Check sheet for the modelled part. Datum: model origin and axes. Units: mm. Round coordinates to 2 decimals unless told otherwise and drop trailing zeros. Order: outer loops, then holes, each group sorted by start corner. A loop starts at its lowest first (then second) coordinate and runs counter-clockwise, first axis right, second up. Notation, with made-up numbers: (17.25, 3.25) -> (41.25, 3.25) arc R13 cw to (41.25, 26.25) -> close; hole circle Ø3 at (16.5, 65.25). An arc over 180 degrees is marked (long way). Answer in a Markdown table with one row per item. Add a question column.
1. Depth check by flat-ended pin: P1, Ø3, axis at x = 75, z = -47, coming from the -Y side; P2, Ø1.1, axis at x = 21, y = 0.5, coming from the +Z side; P3, Ø1.1, axis at y = 0.5, z = -68, coming from the -X side; P4, Ø2.5, axis at x = -7.63, z = 0, coming from the +Y side. Enter the tip coordinate at first touch or a pass-through.
2. Material ranges on L1, parallel to X at y = 0.85, z = 0; L2, parallel to Y at x = 58, z = -13; L3, parallel to X at y = 0.4, z = 32.5, recorded low to high. Write a range as from..to.
3. Sectioned sample at A-A, the plane y = -6.5. Record the boundary of the cut face in (x, z).
4. Sectioned sample at C-C, the plane z = 24. Record the boundary of the cut face in (x, y), then the cut area to 3 significant figures.
5. Sectioned sample at B-B, the plane x = -84. Record the boundary of the cut face in (y, z).
```python
from build123d import *

# Parameters (mm, degrees)
SKETCH1_W            = 208
SKETCH1_H            = 147
BOSS_EXTRUDE1_DEPTH  = 1
CUT_EXTRUDE1_DEPTH   = 128.354819304
MIRROR2_COPY_1_DEPTH = 128.354819304
FILLET1_R            = 10
CUT_EXTRUDE2_DEPTH   = 128.354819304
SKETCH7_R            = 1.5
CUT_EXTRUDE3_DEPTH   = 128.354819304
SKETCH8_R            = 3
BOSS_EXTRUDE3_DEPTH  = 35
SKETCH9_R            = 1.4
CUT_EXTRUDE4_DEPTH   = 60


with BuildPart() as part:
    # Sketch1 → Boss-Extrude1 (new body)
    with BuildSketch(Plane(origin=(0, 0, 0), x_dir=(1, 0, 0), z_dir=(0, 1, 0))):
        Rectangle(SKETCH1_W, SKETCH1_H)
    extrude(amount=BOSS_EXTRUDE1_DEPTH)

    # Sketch3 → Cut-Extrude1 (cut, through all)
    with BuildSketch(Plane(origin=(0, 1, 0), x_dir=(1, 0, 0), z_dir=(0, 1, 0))):
        with BuildLine():
            Line((-89, 83.145473262), (-89, 63.145473262))
            Line((-89, 63.145473262), (-44, 63.145473262))
            Line((-44, 63.145473262), (-44, 58.145473262))
            Line((-44, 58.145473262), (-29, 58.145473262))
            Line((-29, 58.145473262), (-29, 63.145473262))
            Line((-29, 63.145473262), (-14, 63.145473262))
            ThreePointArc((-14, 63.145473262), (-6.928932188, 63.647998579), (0, 65.145473262))
            Line((0, 65.145473262), (0, 85.145473262))
            Line((0, 85.145473262), (-89, 85.145473262))
            Line((-89, 85.145473262), (-89, 83.145473262))
        make_face()
    cut_extrude1 = extrude(amount=-CUT_EXTRUDE1_DEPTH, mode=Mode.SUBTRACT)

    # Mirror1: Cut-Extrude1 across plane
    add(cut_extrude1.mirror(Plane.XY), mode=Mode.SUBTRACT)

    # Mirror2: Cut-Extrude1 across plane
    add(cut_extrude1.mirror(Plane(origin=(0, 0, 0), x_dir=(0, 0, 1), z_dir=(1, 0, 0))), mode=Mode.SUBTRACT)

    # Mirror2 copy 1 sketch → Mirror2 copy 1 (cut, through all)
    with BuildSketch(Plane(origin=(0, 1, 0), x_dir=(-1, 0, 0), z_dir=(0, 1, 0))):
        with BuildLine():
            Line((-89, 83.145473262), (-89, 63.145473262))
            Line((-89, 63.145473262), (-44, 63.145473262))
            Line((-44, 63.145473262), (-44, 58.145473262))
            Line((-44, 58.145473262), (-29, 58.145473262))
            Line((-29, 58.145473262), (-29, 63.145473262))
            Line((-29, 63.145473262), (-14, 63.145473262))
            ThreePointArc((-14, 63.145473262), (-6.928932188, 63.647998579), (0, 65.145473262))
            Line((0, 65.145473262), (0, 85.145473262))
            Line((0, 85.145473262), (-89, 85.145473262))
            Line((-89, 85.145473262), (-89, 83.145473262))
        make_face()
    extrude(amount=-MIRROR2_COPY_1_DEPTH, mode=Mode.SUBTRACT)

    # Fillet1
    fillet1_edges = [part.edges().sort_by_distance(p)[0] for p in [
        (104, 0.5, 73.5),
        (-104, 0.5, 73.5),
        (-104, 0.5, -73.5),
        (104, 0.5, -73.5),
    ]]
    fillet(fillet1_edges, radius=FILLET1_R)

    # Sketch4 → Cut-Extrude2 (cut, through all)
    with BuildSketch(Plane.XZ):
        with BuildLine():
            Line((-58.225796132, 1.876244538), (-49.924870206, 1.876244538))
            ThreePointArc((-49.924870206, 1.876244538), (-49.217763425, 1.583351319), (-48.924870206, 0.876244538))
            Line((-48.924870206, 0.876244538), (-48.924870206, -0.876244538))
            ThreePointArc((-48.924870206, -0.876244538), (-49.217763425, -1.583351319), (-49.924870206, -1.876244538))
            Line((-49.924870206, -1.876244538), (-58.225796132, -1.876244538))
            ThreePointArc((-58.225796132, -1.876244538), (-58.932902913, -2.169137757), (-59.225796132, -2.876244538))
            Line((-59.225796132, -2.876244538), (-59.225796132, -11.176244538))
            ThreePointArc((-59.225796132, -11.176244538), (-59.518689351, -11.883351319), (-60.225796132, -12.176244538))
            Line((-60.225796132, -12.176244538), (-62.62394428, -12.176244538))
            ThreePointArc((-62.62394428, -12.176244538), (-63.331051061, -11.883351319), (-63.62394428, -11.176244538))
            Line((-63.62394428, -11.176244538), (-63.62394428, -2.876244538))
            ThreePointArc((-63.62394428, -2.876244538), (-63.916837499, -2.169137757), (-64.62394428, -1.876244538))
            Line((-64.62394428, -1.876244538), (-72.924870206, -1.876244538))
            ThreePointArc((-72.924870206, -1.876244538), (-73.631976987, -1.583351319), (-73.924870206, -0.876244538))
            Line((-73.924870206, -0.876244538), (-73.924870206, 0.876244538))
            ThreePointArc((-73.924870206, 0.876244538), (-73.631976987, 1.583351319), (-72.924870206, 1.876244538))
            Line((-72.924870206, 1.876244538), (-64.62394428, 1.876244538))
            ThreePointArc((-64.62394428, 1.876244538), (-63.916837499, 2.169137757), (-63.62394428, 2.876244538))
            Line((-63.62394428, 2.876244538), (-63.62394428, 11.823755462))
            ThreePointArc((-63.62394428, 11.823755462), (-63.331051061, 12.530862243), (-62.62394428, 12.823755462))
            Line((-62.62394428, 12.823755462), (-60.225796132, 12.823755462))
            ThreePointArc((-60.225796132, 12.823755462), (-59.518689351, 12.530862243), (-59.225796132, 11.823755462))
            Line((-59.225796132, 11.823755462), (-59.225796132, 2.876244538))
            ThreePointArc((-59.225796132, 2.876244538), (-58.932902913, 2.169137757), (-58.225796132, 1.876244538))
        make_face()
    extrude(amount=-CUT_EXTRUDE2_DEPTH, mode=Mode.SUBTRACT)

    # Sketch7 → Cut-Extrude3 (cut, through all)
    with BuildSketch(Plane.XZ):
        with Locations(Location((43.368968207, 51, 0), (0, 0, 270))):
            Circle(SKETCH7_R)
        with Locations(Location((-7.631031793, 0, 0), (0, 0, 270))):
            Circle(SKETCH7_R)
        with Locations(Location((94.368968207, 0, 0), (0, 0, 270))):
            Circle(SKETCH7_R)
        with Locations(Location((43.368968207, -51, 0), (0, 0, 270))):
            Circle(SKETCH7_R)
    extrude(amount=-CUT_EXTRUDE3_DEPTH, mode=Mode.SUBTRACT)

    # Sketch8 → Boss-Extrude3 (add)
    with BuildSketch(Plane(origin=(0, 1, 0), x_dir=(1, 0, 0), z_dir=(0, 1, 0))):
        with Locations(Location((-95, 65, 0), (0, 0, 270))):
            Circle(SKETCH8_R)
        with Locations(Location((-95, -65, 0), (0, 0, 270))):
            Circle(SKETCH8_R)
        with Locations(Location((97, -65, 0), (0, 0, 270))):
            Circle(SKETCH8_R)
        with Locations(Location((97, 65, 0), (0, 0, 270))):
            Circle(SKETCH8_R)
    extrude(amount=-BOSS_EXTRUDE3_DEPTH)

    # Sketch9 → Cut-Extrude4 (cut)
    with BuildSketch(Plane(origin=(0, 1, 0), x_dir=(1, 0, 0), z_dir=(0, 1, 0))):
        with Locations(Location((-61.740102401, 32.5, 0), (0, 0, 270))):
            Circle(SKETCH9_R)
        with Locations(Location((-94.240102401, 0, 0), (0, 0, 270))):
            Circle(SKETCH9_R)
        with Locations(Location((-61.740102401, -32.5, 0), (0, 0, 270))):
            Circle(SKETCH9_R)
        with Locations(Location((-29.240102401, 0, 0), (0, 0, 270))):
            Circle(SKETCH9_R)
    extrude(amount=-CUT_EXTRUDE4_DEPTH, mode=Mode.SUBTRACT)


solid = part.part
```
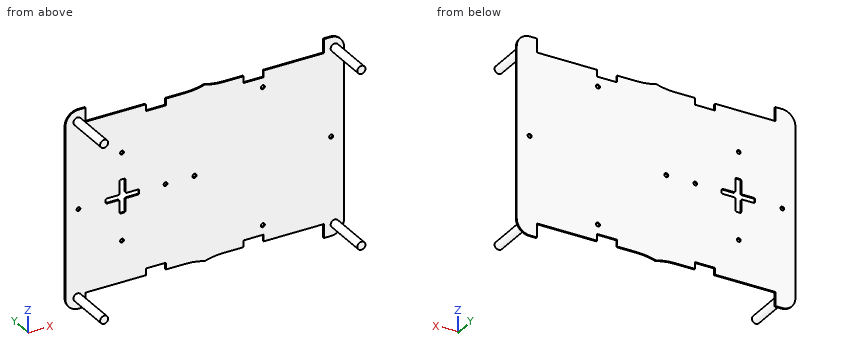
Answer key:
| question | item | result |
|---|---|---|
| 1 | P1 | stops at y = 0 |
| 1 | P2 | stops at z = 63.15 |
| 1 | P3 | stops at x = -103.19 |
| 1 | P4 | passes through |
| 2 | L1 | x = -104..-95.64, -92.84..-73.92, -48.92..-30.64, -27.84..-9.13, -6.13..92.87, 95.87..104 |
| 2 | L2 | y = 0..1 |
| 2 | L3 | x = -104..-63.14, -60.34..104 |
| 3 | outline | circle Ø6 at (-95, -65); circle Ø6 at (-95, 65); circle Ø6 at (97, -65); circle Ø6 at (97, 65) |
| 4 | outline | (-104, 0) -> (104, 0) -> (104, 1) -> (-104, 1) -> close |
| 4 | area | 208 mm² |
| 5 | outline | (0, -63.15) -> (1, -63.15) -> (1, 63.15) -> (0, 63.15) -> close |
